The listing builds one solid part. Answer for the finished solid, in the listing's coordinates (mm). A direction names the side the tool comes from. Coordinates: 2 decimals unless noted, no trailing zeros. Order: outer loops, then holes, each group sorted by start corner. A loop starts at its lowest first (then second) coordinate and runs counter-clockwise, first axis right, second up. Notation, with made-up numbers: (48, 7) -> (67, 7) arc R27 cw to (67, 26) -> close; hole circle Ø2 at (76, 42.5). An arc over 180 degrees is marked (long way). Answer in a Markdown table with one row per item.
```python
from build123d import *

# Parameters (mm, degrees)
F1_DEPTH = 25
F3_DEPTH = 25
F5_DEPTH = 5
F6_R     = 7.5
F7_DEPTH = 20


with BuildPart() as f1:
    # F0 (on Top) → F1 (new body)
    with BuildSketch(Plane.XY):
        with BuildLine():
            Line((45, -20), (45, 20))
            Line((45, 20), (-25, 20))
            ThreePointArc((-25, 20), (-39.142136, 14.142136), (-45, 0))
            ThreePointArc((-45, 0), (-39.142136, -14.142136), (-25, -20))
            Line((-25, -20), (45, -20))
        make_face()
    extrude(amount=F1_DEPTH)

    # F2 (on face) → F3 (cut, through all)
    with BuildSketch(Plane.XY.offset(25)):
        with BuildLine():
            Line((-44.364917, -5), (-33.660254, -5))
            ThreePointArc((-33.660254, -5), (-25, -10), (-16.339746, -5))
            Line((-16.339746, -5), (-10, -5))
            Line((-10, -5), (-10, 5))
            Line((-10, 5), (-16.339746, 5))
            ThreePointArc((-16.339746, 5), (-25, 10), (-33.660254, 5))
            Line((-33.660254, 5), (-44.364917, 5))
            ThreePointArc((-44.364917, 5), (-45, 0), (-44.364917, -5))
        make_face()
    extrude(amount=-F3_DEPTH, mode=Mode.SUBTRACT)

    # F4 (on face) → F5 (cut)
    with BuildSketch(Plane.XY.offset(25)):
        with BuildLine():
            Line((45, -15), (45, 15))
            Line((45, 15), (15, 15))
            ThreePointArc((15, 15), (4.393398, 10.606602), (0, 0))
            ThreePointArc((0, 0), (4.393398, -10.606602), (15, -15))
            Line((15, -15), (45, -15))
        make_face()
    extrude(amount=-F5_DEPTH, mode=Mode.SUBTRACT)

    # F6 (on face) → F7 (cut, through all)
    with BuildSketch(Plane.XY.offset(20)):
        with Locations((15, 0)):
            Circle(F6_R)
    extrude(amount=-F7_DEPTH, mode=Mode.SUBTRACT)


solid = f1.part
```
(1) A cutting plane is placed at D-D, the plane x = 39.5. Determine the outline of the cut face in (y, z).
Check values:
| item | result |
|---|---|
| outline | (-20, 0) -> (20, 0) -> (20, 25) -> (15, 25) -> (15, 20) -> (-15, 20) -> (-15, 25) -> (-20, 25) -> close |
(2) A cutting plane is placed at C-C, the plane y = 9. Determine the outline of the cut face in (x, z).
Check values:
| item | result |
|---|---|
| outline | (-42.86, 0) -> (-29.36, 0) -> (-29.36, 25) -> (-42.86, 25) -> close; (-20.64, 0) -> (45, 0) -> (45, 20) -> (3, 20) -> (3, 25) -> (-20.64, 25) -> close |
(3) A cutting plane is placed at B-B, the plane z = 10.25. Determine the outline of the cut face in (x, y).
Check values:
| item | result |
|---|---|
| outline | (-44.36, -5) arc R20 ccw to (-25, -20) -> (45, -20) -> (45, 20) -> (-25, 20) arc R20 ccw to (-44.36, 5) -> (-33.66, 5) arc R10 cw to (-16.34, 5) -> (-10, 5) -> (-10, -5) -> (-16.34, -5) arc R10 cw to (-33.66, -5) -> close; hole circle Ø15 at (15, 0) |
(4) Find the intervals of material crossed by line 1 along Y through (x, z) = (15, 11.5); line 2 along Y through (x, z) = (-14, 23); line 3 along X through (y, z) = (-8, 5.5), in increasing order. Write a range as from..to.
Check values:
| item | result |
|---|---|
| line 1 | -20..-7.5, 7.5..20 |
| line 2 | -20..-5, 5..20 |
| line 3 | -43.33..-31, -19..45 |
(5) For a pull along Y with two mould halves and no side action, classify faces 4 (the flat face through (-0.3, 0.3, 25)), 5 (the cylindrical face through (-37, -16, 12)), 6 (the flat face through (30, -15, 23)), 7 (the flat face through (10, 20, 12)) as released by +Y, released by -Y, zero draft, split by the parting line, or undercut.
Check values:
| item | result |
|---|---|
| face 4 | zero draft |
| face 5 | released by -Y |
| face 6 | undercut |
| face 7 | released by +Y |
(6) Flat-ended cylindrical pins translate along their axes: pin 1 (2 mm diameter, centred on y = -10, z = 2.5, fed in from -X); pin 2 (9 mm diameter, centred on x = 15, y = 0, fed in from +Z); pin 3 (3 mm diameter, centred on x = -40.5, z = 18, fed in from +Y); pin 4 (8 mm diameter, centred on y = 1.5, z = 16.5, fed in from -X). Find the tip coordinate at first contact, or state that the pin passes through.
Check values:
| item | result |
|---|---|
| pin 1 | x = -42.86 |
| pin 2 | through |
| pin 3 | y = 14.28 |
| pin 4 | x = -44.36 |
(7) A cutting plane is placed at A-A, the plane x = -32.5. Determine the outline of the cut face in (y, z), then the cut area to 3 significant figures.
Check values:
| item | result |
|---|---|
| outline | (-18.54, 0) -> (-6.61, 0) -> (-6.61, 25) -> (-18.54, 25) -> close; (6.61, 0) -> (18.54, 0) -> (18.54, 25) -> (6.61, 25) -> close |
| area | 596 mm² |
(8) Which of the six approach directions +Z, -Z, +X, -X, +Y, -Y give full straight-line access (tool end or side, diameter ignored) to faces 1 (the flat face through (27, 0, 20)), 2 (the cylindrical face through (-25, -10, 13)), 3 (the flat face through (-10, 0, 13))?
Check values:
| item | result |
|---|---|
| face 1 | +Z, +X |
| face 2 | +Z, -Z |
| face 3 | +Z, -Z, -X |
